Geometry check sheet. Reference: the model listing, model coordinates, mm. A direction names the side the tool comes from. Round coordinates to 2 decimals unless told otherwise and drop trailing zeros. Order: outer loops, then holes, each group sorted by start corner. A loop starts at its lowest first (then second) coordinate and runs counter-clockwise, first axis right, second up.
Autodesk Inventor part; units mm, degrees
ref_plane "YZ Plane" through (0, 0, 0) normal (1, 0, 0) x (0, 1, 0)
ref_plane "XZ Plane" through (0, 0, 0) normal (0, 1, 0) x (-1, 0, 0)
ref_plane "XY Plane" through (0, 0, 0) normal (0, 0, 1) x (1, 0, 0)
sketch "Boceto1" plane through (0, 0, 0) normal (0, 0, 1) x (1, 0, 0)
  line L0 (15, -35) -> (-15, -35)
  line L1 (-15, -35) -> (-15, 35)
  line L2 (-15, 35) -> (15, 35)
  line L3 (15, 35) -> (15, -35)
  line L4 (15, -35) -> (-15, 35) construction
  line L5 (-15, -35) -> (15, 35) construction
  line L6 (0, 35) -> (0, -35) construction
  circle A0 centre (0, 28.5) radius 2
  line L7 (-19.7941, 0) -> (22.4931, 0) construction
  circle A1 centre (0, -28.5) radius 2
  point P0 (0, 0)
  dimension "d0" = 70
  dimension "d1" = 30
  dimension "d2" = 4
  dimension "d3" = 6.5
  dimension "d4" = 6.5
extrude "Extrusión1" add sketch "Boceto1" along normal blind 3
sketch "Boceto2" plane through (15, -35, 0) normal (1, 0, 0) x (0, 0, -1)
  line L0 (-1.8712, 18.1097) -> (-14.4034, 50.7658) construction
  line L1 (-14.4034, 50.7658) -> (-23.5228, 61.8317) construction
  line L2 (-23.5228, 61.8317) -> (-35.5227, 59.996) construction
  line L3 (-35.5227, 59.996) -> (-40.0788, 48.4605) construction
  line L4 (-40.0788, 48.4605) -> (-40.0788, 37.855) construction
  line L5 (-40.0788, 37.855) -> (-39.6332, 34.0327) construction
  spline S0 degree 4 poles (-1.8712, 18.1097) (-14.4034, 50.7658) (-23.5228, 61.8317) (-35.5227, 59.996) (-40.0788, 48.4605) (-40.0788, 37.855) (-39.6332, 34.0327) knots 1 1 1 1 1 2 3 4 4 4 4 4 construction
  line L6 (-3, 61.5) -> (-3, 65.5)
  line L7 (-3, 0) -> (-3, 70)
  line L8 (-3, 70) -> (-3, 58)
  line L9 (-3, 58) -> (-27.7071, 61.1916)
  line L10 (-3, 58) -> (-3, 23.1988)
  line L11 (-41.6198, 33.8011) -> (-41.317, 29.2142)
  line L12 (-41.317, 29.2142) -> (-37.8007, 35.959)
  arc A0 (-3, 23.1988) -> (-31.2114, 56.3416) centre (-45.8049, 15.3413) ccw
  spline S1 degree 5 poles (-27.7071, 61.1916) (-28.3861, 61.204) (-29.0661, 61.164) (-29.7416, 61.0697) (-31.212, 60.7437) (-32.6066, 60.1691) (-33.3389, 59.7849) (-34.7268, 58.894) (-35.9529, 57.791) (-36.5222, 57.195) (-37.5948, 55.9044) (-38.4921, 54.486) (-38.9051, 53.737) (-39.672, 52.1477) (-40.273, 50.4882) (-40.5424, 49.6188) (-41.0222, 47.8089) (-41.3636, 45.9678) (-41.5068, 45.0158) (-41.7361, 43.0961) (-41.8573, 41.1666) (-41.8931, 40.1963) (-41.9162, 38.3325) (-41.8502, 36.4697) (-41.7977, 35.5781) (-41.7231, 34.688) (-41.6198, 33.8011) knots 0 0 0 0 0 0 0.098265 0.098265 0.098265 0.217274 0.217274 0.217274 0.336121 0.336121 0.336121 0.459615 0.459615 0.459615 0.591158 0.591158 0.591158 0.730365 0.730365 0.730365 0.870803 0.870803 0.870803 1 1 1 1 1 1
  spline S2 degree 5 poles (-31.2114, 56.3416) (-31.6636, 56.0965) (-32.095, 55.8132) (-32.503, 55.497) (-33.3156, 54.7706) (-34.0235, 53.9412) (-34.3681, 53.4813) (-35.0445, 52.4631) (-35.6063, 51.3769) (-35.8744, 50.7865) (-36.3876, 49.5038) (-36.7878, 48.1811) (-36.9721, 47.4711) (-37.3065, 45.9717) (-37.5429, 44.4536) (-37.643, 43.6569) (-37.8023, 42.0438) (-37.8811, 40.4248) (-37.9018, 39.607) (-37.9054, 38.386) (-37.8672, 37.1658) (-37.85, 36.7633) (-37.8279, 36.3609) (-37.8007, 35.959) knots 0 0 0 0 0 0 0.114517 0.114517 0.114517 0.242166 0.242166 0.242166 0.386331 0.386331 0.386331 0.549516 0.549516 0.549516 0.72821 0.72821 0.72821 0.910298 0.910298 0.910298 1 1 1 1 1 1
  point P0 (0, 35)
  point P1 (-17.4487, 48.3553)
  point P2 (-3, 11.1175)
  point P3 (-18.9631, 49.5979)
  dimension "d7" = 2
  dimension "d9" = 12
  dimension "d10" = 24.7071
  dimension "d32" = 34.8012
  dimension "d33" = 12.0812
  dimension "d34" = 9.1194
  dimension "d35" = 11.0659
  dimension "d36" = 32.6561
  dimension "d37" = 12.5322
  dimension "d38" = 43.5201
  dimension "d39" = 10.6055
  dimension "d40" = 3.5163
  dimension "d41" = 6.7448
  dimension "d42" = 34.8008
  dimension "d43" = 20.3826
  dimension "d44" = 1.6584
  dimension "d45" = 16.556
  dimension "d46" = 13.3712
extrude "Extrusión2" add sketch "Boceto2" against normal up to surface (30 mm away)
fillet "Empalme5" radius 10 1 edges at (0, 21.3416, 31.2114)
fillet "Empalme6" radius 1 1 edges at (0, -5.7858, 41.317)
sketch "Boceto3" plane through (15, -35, 0) normal (1, 0, 0) x (0, 0, -1)
  arc A0 (-41.552, 32.7748) -> (-39.6675, 32.3783) centre (-40.5542, 32.8406) ccw
  line L0 (-39.6675, 32.3783) -> (-37.8007, 35.959)
  spline S0 degree 5 poles (-37.8007, 35.959) (-37.8279, 36.3609) (-37.85, 36.7633) (-37.8672, 37.1658) (-37.9054, 38.386) (-37.9018, 39.607) (-37.8811, 40.4248) (-37.8125, 41.8353) (-37.6827, 43.2413) (-37.6167, 43.8317) (-37.5385, 44.4206) (-37.4469, 45.0073) knots 0 0 0 0 0 0 0.222024 0.222024 0.222024 0.672714 0.672714 0.672714 1 1 1 1 1 1
  spline S1 degree 2 poles (-22.1255, 51.8554) (-35.0681, 60.2487) (-37.4469, 45.0073) knots 0 0 0 1 1 1 weights 1 0.543962 1
  arc A1 (-3, 23.1988) -> (-22.1255, 51.8554) centre (-45.8049, 15.3413) ccw
  line L1 (-3, 0) -> (-3, 23.1988)
  line L2 (0, 0) -> (-3, 0)
  line L3 (0, 70) -> (0, 0)
  line L4 (0, 70) -> (-3, 70)
  line L5 (-3, 58) -> (-3, 70)
  line L6 (-3, 58) -> (-27.7071, 61.1916)
  spline S2 degree 5 poles (-27.7071, 61.1916) (-28.3861, 61.204) (-29.0661, 61.164) (-29.7416, 61.0697) (-31.212, 60.7437) (-32.6066, 60.1691) (-33.3389, 59.7849) (-34.7268, 58.894) (-35.9529, 57.791) (-36.5222, 57.195) (-37.5948, 55.9044) (-38.4921, 54.486) (-38.9051, 53.737) (-39.672, 52.1477) (-40.273, 50.4882) (-40.5424, 49.6188) (-41.0222, 47.8089) (-41.3636, 45.9678) (-41.5068, 45.0158) (-41.7361, 43.0961) (-41.8573, 41.1666) (-41.8931, 40.1963) (-41.9162, 38.3325) (-41.8502, 36.4697) (-41.7977, 35.5781) (-41.7231, 34.688) (-41.6198, 33.8011) knots 0 0 0 0 0 0 0.098265 0.098265 0.098265 0.217274 0.217274 0.217274 0.336121 0.336121 0.336121 0.459615 0.459615 0.459615 0.591158 0.591158 0.591158 0.730365 0.730365 0.730365 0.870803 0.870803 0.870803 1 1 1 1 1 1
  line L7 (-41.6198, 33.8011) -> (-41.552, 32.7748)
  line L8 (-3, 58) -> (-3, 23.1988)
  point P0 (0, 35)
extrude "Extrusión3" cut sketch "Boceto3" against normal blind 6 contours L7 S2 L6 L8 A1 S1 S0 L0 A0
sketch "Boceto4" plane through (-15, -35, 0) normal (-1, 0, 0) x (0, 0, 1)
  arc A0 (41.552, 32.7748) -> (39.6675, 32.3783) centre (40.5542, 32.8406) ccw
  line L0 (41.6198, 33.8011) -> (41.552, 32.7748)
  spline S0 degree 3 poles (27.7071, 61.1916) (29.0874, 61.2167) (30.4423, 60.9813) (33.0627, 59.9896) (34.2716, 59.2392) (36.6603, 57.1563) (37.7384, 55.7597) (39.8454, 52.037) (40.6354, 49.5891) (42.0928, 42.3499) (42.0185, 37.2222) (41.6198, 33.8011) knots 0 0 0 0 0.414156 0.414156 0.839985 0.839985 1.363183 1.363183 2.115437 2.115437 3.566985 3.566985 3.566985 3.566985
  line L1 (3, 58) -> (27.7071, 61.1916)
  arc A1 (22.1255, 51.8554) -> (3, 23.1988) centre (45.8049, 15.3413) ccw
  spline S1 degree 3 poles (37.4469, 45.0073) (37.2461, 46.2939) (36.7959, 47.529) (35.4475, 49.757) (34.5621, 50.7287) (32.4688, 52.2779) (31.2808, 52.8407) (28.756, 53.4793) (27.4433, 53.5489) (25.4381, 53.2629) (24.7351, 53.0833) (23.3803, 52.5756) (22.7324, 52.2491) (22.1255, 51.8554) knots 0 0 0 0 0.390644 0.390644 0.781289 0.781289 1.171933 1.171933 1.562578 1.562578 1.779598 1.779598 1.996619 1.996619 1.996619 1.996619
  spline S2 degree 3 poles (37.8007, 35.959) (37.9656, 38.3979) (37.96, 41.7196) (37.4469, 45.0073) knots 0 0 0 0 0.733359 0.733359 0.733359 0.733359
  line L2 (39.6675, 32.3783) -> (37.8007, 35.959)
  line L3 (3, 58) -> (3, 23.1988)
  line L4 (3, 58) -> (3, 23.1988)
  arc A2 (41.552, 32.7748) -> (39.6675, 32.3783) centre (40.5542, 32.8406) ccw
  line L5 (41.6198, 33.8011) -> (41.552, 32.7748)
  spline S3 degree 3 poles (27.7071, 61.1916) (29.0874, 61.2167) (30.4423, 60.9813) (33.0627, 59.9896) (34.2716, 59.2392) (36.6603, 57.1563) (37.7384, 55.7597) (39.8454, 52.037) (40.6354, 49.5891) (42.0928, 42.3499) (42.0185, 37.2222) (41.6198, 33.8011) knots 0 0 0 0 0.414156 0.414156 0.839985 0.839985 1.363183 1.363183 2.115437 2.115437 3.566985 3.566985 3.566985 3.566985
  line L6 (3, 58) -> (27.7071, 61.1916)
  arc A3 (22.1255, 51.8554) -> (3, 23.1988) centre (45.8049, 15.3413) ccw
  spline S4 degree 3 poles (37.4469, 45.0073) (37.2461, 46.2939) (36.7959, 47.529) (35.4475, 49.757) (34.5621, 50.7287) (32.4688, 52.2779) (31.2808, 52.8407) (28.756, 53.4793) (27.4433, 53.5489) (25.4381, 53.2629) (24.7351, 53.0833) (23.3803, 52.5756) (22.7324, 52.2491) (22.1255, 51.8554) knots 0 0 0 0 0.390644 0.390644 0.781289 0.781289 1.171933 1.171933 1.562578 1.562578 1.779598 1.779598 1.996619 1.996619 1.996619 1.996619
  spline S5 degree 3 poles (37.8007, 35.959) (37.9656, 38.3979) (37.96, 41.7196) (37.4469, 45.0073) knots 0 0 0 0 0.733359 0.733359 0.733359 0.733359
  line L7 (39.6675, 32.3783) -> (37.8007, 35.959)
  circle A4 centre (40.5542, 32.8406) radius 1
  point P0 (0, 35)
extrude "Extrusión4" cut sketch "Boceto4" against normal blind 6
sketch "Boceto5" plane through (0, 0, 3) normal (0, 0, 1) x (1, 0, 0)
  circle A0 centre (0, -28.5) radius 2
  circle A1 centre (0, -28.5) radius 4.6184
  circle A2 centre (0, 28.5) radius 2
  circle A3 centre (0, 28.5) radius 3.6227
  point P0 (0, 0)
extrude "Extrusión5" add sketch "Boceto5" against normal up to surface (3 mm away) contours A0 | A2
sketch "Boceto6" plane through (0, 0, 3) normal (0, 0, 1) x (1, 0, 0)
  circle A0 centre (0, -19.7984) radius 2.1
  line L0 (-14.9492, 6.775) -> (15, 6.775) construction
  line L1 (15, -35) -> (15, 35)
  line L2 (11, 25.275) -> (-11, 25.275)
  line L3 (9, -11.8012) -> (-9, -11.8012)
  circle A1 centre (0, 33.3483) radius 2.1
  line L4 (-15, -35) -> (15, -35)
  line L5 (-15, 35) -> (-15, -35)
  point P0 (0, 0)
  point P1 (11, -11.8012)
  point P2 (-11, -11.8012)
  dimension "d66" = 4.2
  dimension "d67" = 15.2016
  dimension "d68" = 15
sketch "Boceto7" plane through (0, 0, 3) normal (0, 0, 1) x (1, 0, 0)
  line L0 (-15, -35) -> (15, -35)
  line L1 (15, -35) -> (15, 35)
  line L2 (-15, -35) -> (15, -35)
  line L3 (15, -35) -> (15, -29.7984)
  line L4 (15, -29.7984) -> (-15, -29.7984)
  line L5 (-15, -29.7984) -> (-15, -35)
  circle A0 centre (0, -19.7984) radius 2.1
  point P0 (0, 0)
  dimension "d51" = 10
extrude "Extrusión6" cut sketch "Boceto7" against normal blind 7 contours L5 L4 L1 L0
sketch "Boceto8" plane through (0, 0, 3) normal (0, 0, 1) x (1, 0, 0)
  line L0 (-15, 35) -> (15, 35)
  line L1 (15, 35) -> (15, 43.3483)
  line L2 (15, 43.3483) -> (-15, 43.3483)
  line L3 (-15, 43.3483) -> (-15, 35)
  circle A0 centre (0, 33.3483) radius 2.1
  point P0 (0, 0)
  dimension "d54" = 10
extrude "Extrusión7" add sketch "Boceto8" against normal up to surface (3 mm away) contours L3 L2 L1 L0 A0 | A0 L0 picked at (-0.3005, 35.0816)
sketch "Boceto9" plane through (0, 0, 3) normal (0, 0, 1) x (1, 0, 0)
  line L0 (15, 43.3483) -> (-15, 43.3483)
  line L1 (9, -29.7984) -> (9, 43.3483)
  line L2 (-9, 43.3483) -> (-9, -29.7984)
  line L3 (-15, -29.7984) -> (15, -29.7984)
  line L4 (-9, -11.8012) -> (-9, 23)
  line L5 (9, 23) -> (9, -11.8012)
  line L6 (-15, 43.3483) -> (-15, -29.7984)
  line L7 (-9, -29.7984) -> (-15, -29.7984)
  line L8 (-15, -29.7984) -> (-15, 43.3483)
  line L9 (-15, 43.3483) -> (-9, 43.3483)
  line L10 (-9, 43.3483) -> (-9, -29.7984)
  line L11 (15, -29.7984) -> (15, 43.3483)
  line L12 (9, 43.3483) -> (15, 43.3483)
  line L13 (15, 43.3483) -> (15, -29.7984)
  line L14 (15, -29.7984) -> (9, -29.7984)
  line L15 (9, -29.7984) -> (9, 43.3483)
  point P0 (0, 0)
extrude "Extrusión8" cut sketch "Boceto9" against normal blind 7 contours L11 L3 L1 L0 | L2 L3 L6 L0
sketch "Boceto10" plane through (0, 0, 0) normal (0, 0, -1) x (-1, 0, 0)
  line L0 (9, 43.3483) -> (9, 23)
  line L1 (-9, -29.7984) -> (-9, -11.8012)
  line L2 (9, 43.3483) -> (-9, 43.3483)
  line L3 (-9, 43.3483) -> (-9, -29.7984)
  line L4 (-9, -29.7984) -> (9, -29.7984)
  line L5 (9, -29.7984) -> (9, 43.3483)
  point P0 (0, 0)
extrude "Extrusión9" add sketch "Boceto10" along normal blind 1
extrude "Extrusión10" cut sketch "Boceto6" against normal up to surface (4 mm away)
chamfer "Chaflán1" distance 1 angle 45 2 edges at (-2.1, -19.7984, 3) (-2.1, 33.3483, 3)
fillet "Empalme8" radius 5 1 edges at (0, 23, 3)
equation "\"d4\" = d3"
properties part number "CoronaVirus"
(1) Depth check by flat-ended pin: P1, Ø4, axis at x = 0, y = 33.35, coming from the -Z side; P2, Ø6, axis at x = -5.5, z = 11.5, coming from the +Y side; P3, Ø6, axis at x = 7, z = 25.5, coming from the -Y side; P4, Ø5.5, axis at x = -1, y = -24, coming from the +Z side. Enter the tip coordinate at first touch or a pass-through.
Returned:
P1: passes through
P2: stops at y = 24.49
P3: stops at y = 17.09
P4: stops at z = 3
(2) Material ranges on line 1 (Y direction, x = 0, z = -0.15); line 2 (Z direction, x = 3.25, y = 40); line 3 (Z direction, x = -5.25, y = 21), recorded low to high.
Returned:
line 1: y = -29.8 to -21.9, -17.7 to 31.25, 35.45 to 43.35
line 2: z = -1 to 3
line 3: z = -1 to 37.46
(3) Draft check along Y on faces 5 (the cylindrical face through (-0.27, 35.43, 0.52)), 6 (the cylindrical face through (-0.455, -21.848, 0.521)), 7 (the cylindrical face through (-0.126, 24.972, 4.654)), 8 (the flat face through (0, 7, -1)). Enter one of: released by +Y, released by -Y, zero draft, split by the parting line, or undercut.
Returned:
face 5: undercut
face 6: undercut
face 7: released by +Y
face 8: zero draft
(4) Sectioned sample at B-B, the plane y = -9.5. Record the cut outline in (x, z).
Returned:
outline: (-9, -1) - (9, -1) - (9, 3.49) - (-9, 3.49) - close
(5) Sectioned sample at C-C, the plane z = 4. Record the cut outline in (x, y), and give its area (3 significant figures).
Returned:
outline: (-9, -7.56) - (9, -7.56) - (9, 25.69) - (-9, 25.69) - close
area: 598 mm2
(6) Set-up check for faces 1 (the flat face through (-2, -23, 3)), 2 (the flat face through (0, 38, 3)), 3 (the flat face through (0.13, -0.86, 38.75)), 4 (the flat face through (0.126, 24.943, 18.04)): record each of +Z, -Z, +X, -X, +Y, -Y from which the full face is reachable in a straight line by a thin tool's end or side.
Returned:
face 1: +Z, +X, -X, -Y
face 2: +Z, +X, -X, +Y
face 3: +X, -X, -Y
face 4: +X, -X, +Y
(7) Sectioned sample at A-A, the plane x = 0. Give the number of separate pieces and of enclosed holes in the cut face, and give its area (3 significant figures).
Returned:
separate pieces: 3
enclosed holes: 0
area: 797 mm2
